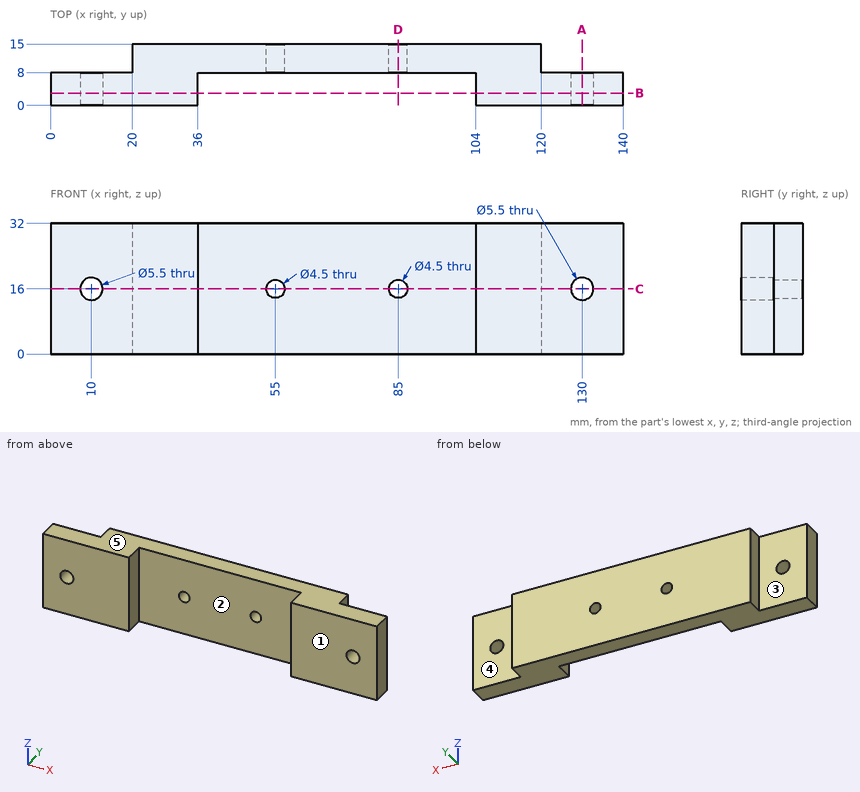
Geometry check sheet. Reference: drawing and pictorial views, mm from the part's lowest x, y, z. A direction names the side the tool comes from. Coordinates: 2 decimals unless noted, no trailing zeros. Order: outer loops, then holes, each group sorted by start corner. A loop starts at its lowest first (then second) coordinate and runs counter-clockwise, first axis right, second up.
Item 1: Section check C-C (z = 16). Enter the section's corners in (x, y).
Item 2: Tool access check on the marked faces 3, 4 and 5. Record the directions out of +Z, -Z, +X, -X, +Y, -Y that give a thin tool (end or side, any length) a straight path to the whole face; none if there is none.
Item 3: Section check B-B (y = 3). Enter the section's corners in (x, z), plus the area to 3 significant figures.
Item 4: Section check D-D (x = 85). Enter the section's corners in (y, z).
Item 5: Section check A-A (x = 130). Enter the section's corners in (y, z).
Item 6: Mould release check, pull along X, two halves, no side actions. Record for the marked faces 1 and 2: released by +X, released by -X, zero draft, split by the parting line, or undercut.
Item 7: Depth check by flat-ended pin: pin 1 (9 mm diameter, centred on x = 130, z = 16, fed in from +Y); pin 2 (3.5 mm diameter, centred on x = 55, z = 16, fed in from +Y); pin 3 (2 mm diameter, centred on y = 12.5, z = 8.5, fed in from +X). Enter the tip coordinate at first touch or a pass-through.
Item 8: Scan lines: line 1 along X through (y, z) = (10.5, 16); line 2 along X through (y, z) = (3.25, 16); line 3 along Z through (x, y) = (130, 6). Record each from-to range of solid material in increasing order.
Check sheet entries:
1. outline: (0, 0) - (7.25, 0) - (7.25, 8) - (0, 8) - close; (12.75, 0) - (36, 0) - (36, 8) - (52.75, 8) - (52.75, 15) - (20, 15) - (20, 8) - (12.75, 8) - close; (57.25, 8) - (82.75, 8) - (82.75, 15) - (57.25, 15) - close; (87.25, 8) - (104, 8) - (104, 0) - (127.25, 0) - (127.25, 8) - (120, 8) - (120, 15) - (87.25, 15) - close; (132.75, 0) - (140, 0) - (140, 8) - (132.75, 8) - close
2. face 3: +Z, -Z, -X, +Y
2. face 4: +Z, -Z, +X, +Y
2. face 5: +Z, +X, -X, +Y, -Y
3. outline: (0, 0) - (36, 0) - (36, 32) - (0, 32) - close; (104, 0) - (140, 0) - (140, 32) - (104, 32) - close; hole circle Ø5.5 at (10, 16); hole circle Ø5.5 at (130, 16)
3. area: 2,260 mm2
4. outline: (8, 0) - (15, 0) - (15, 13.75) - (8, 13.75) - close; (8, 18.25) - (15, 18.25) - (15, 32) - (8, 32) - close
5. outline: (0, 0) - (8, 0) - (8, 13.25) - (0, 13.25) - close; (0, 18.75) - (8, 18.75) - (8, 32) - (0, 32) - close
6. face 1: zero draft
6. face 2: undercut
7. pin 1: stops at y = 8
7. pin 2: passes through
7. pin 3: stops at x = 120
8. line 1: x = 20 to 52.75, 57.25 to 82.75, 87.25 to 120
8. line 2: x = 0 to 7.25, 12.75 to 36, 104 to 127.25, 132.75 to 140
8. line 3: z = 0 to 13.25, 18.75 to 32
